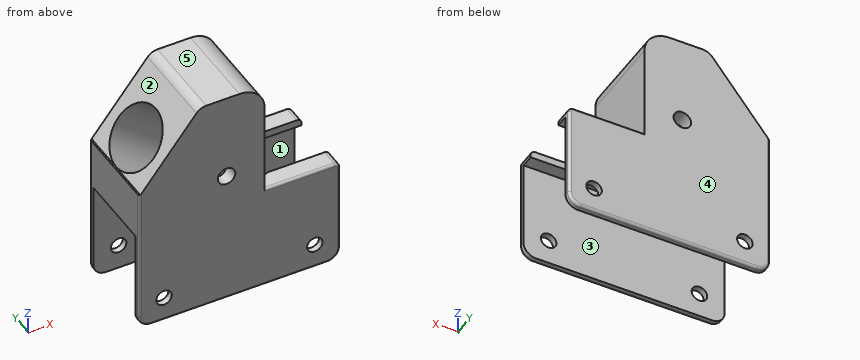
from build123d import *

# Parameters (mm, degrees)
F0_R      = 3.1
F1_DEPTH  = 17.6
F2_W      = 80
F2_H      = 40
F3_DEPTH  = 15.1
F4_R      = 5
F5_R      = 5
F6_R      = 10
F8_DEPTH  = 5
F9_R      = 12.75
F10_DEPTH = 99.501459
F11_R     = 2
F12_R     = 1
F13_R     = 3.5
F14_DEPTH = 40


with BuildPart() as f1:
    # F0 (on Front) → F1 (new body, symmetric)
    with BuildSketch(Plane.XZ):
        with BuildLine():
            Line((-40, -21.5), (40, -21.5))
            Line((40, -21.5), (40, 21.5))
            Line((40, 21.5), (10, 21.5))
            Line((10, 21.5), (10, 68.5))
            Line((10, 68.5), (-13.177477, 68.5))
            ThreePointArc((-13.177477, 68.5), (-15.35175, 68.002504), (-17.093345, 66.609015))
            Line((-17.093345, 66.609015), (-39.385551, 38.531528))
            Line((-39.385551, 38.531528), (-39.330944, 38.5))
            Line((-39.330944, 38.5), (-40, 38.5))
            Line((-40, 38.5), (-40, 21.5))
            Line((-40, 21.5), (-40, -21.5))
        make_face()
        with Locations((-30, -11.5)):
            Circle(F0_R, mode=Mode.SUBTRACT)
        with Locations((30, -11.5)):
            Circle(F0_R, mode=Mode.SUBTRACT)
    extrude(amount=F1_DEPTH, both=True)

    # F2 (on Front) → F3 (cut, symmetric)
    with BuildSketch(Plane.XZ):
        with Locations((0, -1.5)):
            Rectangle(F2_W, F2_H)
    extrude(amount=F3_DEPTH, both=True, mode=Mode.SUBTRACT)

    # F4
    f4_edges = [f1.edges().sort_by_distance(p)[0] for p in [
        (40, 16.35, -21.5),
        (40, -16.35, -21.5),
    ]]
    fillet(f4_edges, radius=F4_R)

    # F5
    f5_edges = [f1.edges().sort_by_distance(p)[0] for p in [
        (-40, 16.35, -21.5),
        (-40, -16.35, -21.5),
    ]]
    fillet(f5_edges, radius=F5_R)

    # F6
    f6_edges = [f1.edges().sort_by_distance(p)[0] for p in [
        (10, 0, 68.5),
    ]]
    fillet(f6_edges, radius=F6_R)

    # F7 (on face) → F8 (cut)
    with BuildSketch(Plane.XY.offset(21.5)):
        with BuildLine():
            Line((15, -10), (40, -10))
            Line((40, -10), (40, 0))
            Line((40, 0), (40, 10))
            Line((40, 10), (15, 10))
            ThreePointArc((15, 10), (11.464466, 8.535534), (10, 5))
            Line((10, 5), (10, -5))
            ThreePointArc((10, -5), (11.464466, -8.535534), (15, -10))
        make_face()
    extrude(amount=-F8_DEPTH, mode=Mode.SUBTRACT)

    # F9 (on face) → F10 (cut, through all)
    with BuildSketch(Plane(origin=(-42.921633, 0, 34.07776), x_dir=(0, -1, 0), z_dir=(-0.783174, 0, 0.621803))):
        with Locations((0, 18.526129)):
            Circle(F9_R)
    extrude(amount=-F10_DEPTH, mode=Mode.SUBTRACT)

    # F11
    f11_edges = [f1.edges().sort_by_distance(p)[0] for p in [
        (40, 13.8, 21.5),
        (40, -13.8, 21.5),
    ]]
    fillet(f11_edges, radius=F11_R)

    # F12
    f12_edges = [f1.edges().sort_by_distance(p)[0] for p in [
        (40, -17.6, 1.5),
        (40, 17.6, 1.5),
    ]]
    fillet(f12_edges, radius=F12_R)

    # F13 (on face) → F14 (cut)
    with BuildSketch(Plane.XZ.offset(17.6)):
        with Locations((-5.136279, 33.422398)):
            Circle(F13_R)
    extrude(amount=-F14_DEPTH, mode=Mode.SUBTRACT)


solid = f1.part
Part model, mm, in its own coordinate system. Face numbers are marked on the shaded views. A direction names the side the tool comes from. Coordinates: 2 decimals unless noted, no trailing zeros. Loops run counter-clockwise (first coordinate to the right, second up) from the corner with the lowest first, then second, coordinate; pieces in that order, holes last. Notation, with made-up numbers: (-28, -2) - (-10, -2) arc R19 cw to (-10, 4) - close; hole circle Ø7 at (-2, 72.25). An arc over 180 degrees is marked (long way). Write each question's results on one line, items separated by ' | '. Start each with the question number.
Q1. Two-plate mould, pull along Y, no slides. Class the marked faces 3, 4 and 5: +Y half, -Y half, draft (parallel to the pull), parting line (faces both ways), or undercut.
Q2. Drop flat-ended pins along their axis: pin 1 Ø0.7 at (x, y) = (-39.5, 1.5) entering from +Z; pin 2 Ø3 at (y, z) = (10, 54.5) entering from +X; pin 3 Ø7.5 at (x, y) = (23, -13) entering from +Z; pin 4 Ø6 at (x, z) = (-28, 59) entering from -Y. Give the stop position or say it passes through.
Q3. Slice it at B-B on z = 14. Give the cut face in (x, y).
Q4. Which spindle directions (+Z, -Z, +X, -X, +Y, -Y) get a long thin tool onto all of the face, cutting with end or side? Do the marked faces 1 and 2. Say none if no direction does.
Q5. Slice it at A-A on x = 30. Give the cut face in (y, z), and give its area (3 significant figures).
Q6. Slice it at C-C on z = -11.5. Give the cut face in (x, y), and give its area (3 significant figures).
Q7. Probe line 1 along X through (y, z) = (16.15, -11.5); line 2 along Y through (x, z) = (36, -15); line 3 along Z through (x, y) = (30, 16.2). List the from-to ranges inside material, lowest first.
Q8. Slice it at D-D on y = -5.5. Give the cut face in (x, z), and give its area (3 significant figures).
Answer:
1) face 3: undercut | face 4: +Y half | face 5: draft
2) pin 1: stops at z = 38.7 | pin 2: stops at x = 10 | pin 3: stops at z = 21.5 | pin 4: passes through
3) outline: (-40, -16.6) arc R1 ccw to (-39, -17.6) - (39, -17.6) arc R1 ccw to (40, -16.6) - (40, -15.1) - (-40, -15.1) - close; (-40, 15.1) - (40, 15.1) - (40, 16.6) arc R1 ccw to (39, 17.6) - (-39, 17.6) arc R1 ccw to (-40, 16.6) - close
4) face 1: -Z, +X, -X | face 2: +Z, -X, +Y, -Y
5) outline: (-17.6, -20.5) arc R1 ccw to (-16.6, -21.5) - (-15.1, -21.5) - (-15.1, -14.6) - (-17.6, -14.6) - close; (-17.6, -8.4) - (-15.1, -8.4) - (-15.1, 18.5) - (-10, 18.5) - (-10, 21.5) - (-16.6, 21.5) arc R1 ccw to (-17.6, 20.5) - close; (10, 18.5) - (15.1, 18.5) - (15.1, -8.4) - (17.6, -8.4) - (17.6, 20.5) arc R1 ccw to (16.6, 21.5) - (10, 21.5) - close; (15.1, -21.5) - (16.6, -21.5) arc R1 ccw to (17.6, -20.5) - (17.6, -14.6) - (15.1, -14.6) - close | area: 214 mm2
6) outline: (-40, -16.6) arc R1 ccw to (-39, -17.6) - (-33.1, -17.6) - (-33.1, -15.1) - (-40, -15.1) - close; (-40, 15.1) - (-33.1, 15.1) - (-33.1, 17.6) - (-39, 17.6) arc R1 ccw to (-40, 16.6) - close; (-26.9, -17.6) - (26.9, -17.6) - (26.9, -15.1) - (-26.9, -15.1) - close; (-26.9, 15.1) - (26.9, 15.1) - (26.9, 17.6) - (-26.9, 17.6) - close; (33.1, -17.6) - (39, -17.6) arc R1 ccw to (40, -16.6) - (40, -15.1) - (33.1, -15.1) - close; (33.1, 15.1) - (40, 15.1) - (40, 16.6) arc R1 ccw to (39, 17.6) - (33.1, 17.6) - close | area: 337 mm2
7) line 1: x = -40 to -33.1, -26.9 to 26.9, 33.1 to 40 | line 2: y = -17.6 to -15.1, 15.1 to 17.6 | line 3: z = -21.5 to -14.6, -8.4 to 21.5
8) outline: (-40, 18.5) - (-12.01, 18.5) - (-38.55, 39.58) - (-39.39, 38.53) - (-39.33, 38.5) - (-40, 38.5) - close; (-24.25, 57.6) - (10, 30.4) - (10, 58.5) arc R10 ccw to (0, 68.5) - (-13.18, 68.5) arc R5 ccw to (-17.09, 66.61) - close | area: 1,080 mm2
